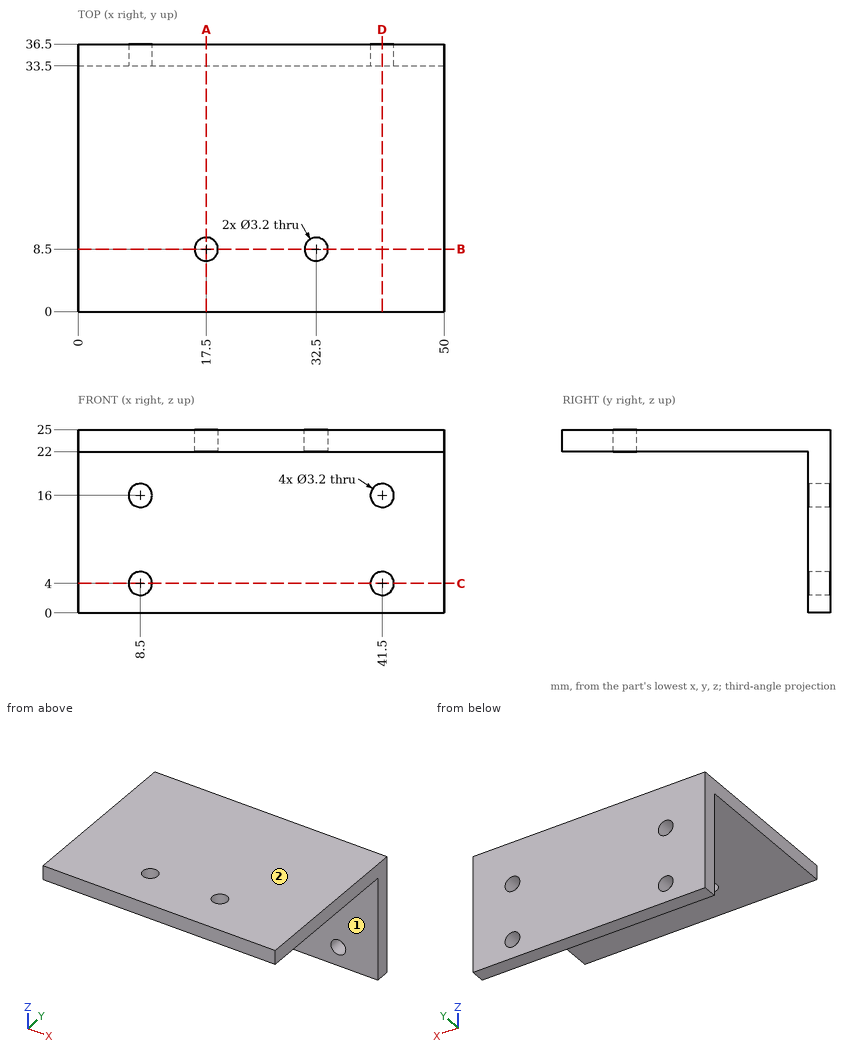
For this review, use the dimensioned drawing (mm, ordinates from the lowest corner) and the shaded views. A direction names the side the tool comes from. Round coordinates to 2 decimals unless told otherwise and drop trailing zeros. Order: outer loops, then holes, each group sorted by start corner. A loop starts at its lowest first (then second) coordinate and runs counter-clockwise, first axis right, second up. Notation, with made-up numbers: (1.25, 47.25) -> (9.25, 47.25) arc R17 cw to (9.25, 77.25) -> close; hole circle Ø6 at (-13, 60.25). An arc over 180 degrees is marked (long way). One line per item, written item: value. Start each with the question number.
Q1. Take a section at D-D (x = 41.5). Write out the cut boundary in (y, z), and give its area (3 significant figures).
Q2. Wall thickness on line 1 (Z direction, x = 8.5, y = 35.65); line 2 (Z direction, x = 45, y = 9); line 3 (Y direction, x = 30.5, z = 1.5): over which ranges is each line inside the solid? List them lowest first.
Q3. Clearance check with flat-ended pins moving along their axes: pin 1 Ø10 at (y, z) = (10, 18.5) entering from +X; pin 2 Ø3.5 at (x, y) = (32.5, 8.5) entering from -Z; pin 3 Ø5 at (x, z) = (41.5, 4) entering from -Y. State where each tip first meets the part, or that it passes through.
Q4. Machinability: for the marked faces 1 and 2, which of the approach directions +Z, -Z, +X, -X, +Y, -Y give a long, thin tool a straight path to every point of the face, cutting with its end or side? Answer none if there is none.
Q5. Take a section at C-C (z = 4). Write out the cut boundary in (x, y), and give its area (3 significant figures).
Q6. Take a section at B-B (y = 8.5). Write out the cut boundary in (x, z).
Q7. Take a section at A-A (x = 17.5). Write out the cut boundary in (y, z).
Reported:
1. outline: (0, 22) -> (33.5, 22) -> (33.5, 17.6) -> (36.5, 17.6) -> (36.5, 25) -> (0, 25) -> close; (33.5, 0) -> (36.5, 0) -> (36.5, 2.4) -> (33.5, 2.4) -> close; (33.5, 5.6) -> (36.5, 5.6) -> (36.5, 14.4) -> (33.5, 14.4) -> close
1. area: 156 mm2
2. line 1: z = 0 to 2.4, 5.6 to 14.4, 17.6 to 25
2. line 2: z = 22 to 25
2. line 3: y = 33.5 to 36.5
3. pin 1: stops at x = 50
3. pin 2: stops at z = 22
3. pin 3: stops at y = 33.5
4. face 1: -Z, +X, -X, -Y
4. face 2: +Z, +X, -X, +Y, -Y
5. outline: (0, 33.5) -> (6.9, 33.5) -> (6.9, 36.5) -> (0, 36.5) -> close; (10.1, 33.5) -> (39.9, 33.5) -> (39.9, 36.5) -> (10.1, 36.5) -> close; (43.1, 33.5) -> (50, 33.5) -> (50, 36.5) -> (43.1, 36.5) -> close
5. area: 131 mm2
6. outline: (0, 22) -> (15.9, 22) -> (15.9, 25) -> (0, 25) -> close; (19.1, 22) -> (30.9, 22) -> (30.9, 25) -> (19.1, 25) -> close; (34.1, 22) -> (50, 22) -> (50, 25) -> (34.1, 25) -> close
7. outline: (0, 22) -> (6.9, 22) -> (6.9, 25) -> (0, 25) -> close; (10.1, 22) -> (33.5, 22) -> (33.5, 0) -> (36.5, 0) -> (36.5, 25) -> (10.1, 25) -> close
